For this review, use the dimensioned drawing (mm, ordinates from the lowest corner) and the shaded views. Round coordinates to 2 decimals unless told otherwise and drop trailing zeros. Write each loop counter-clockwise with the first axis right and the second up, starting at its lowest first coordinate (ties: lowest second). Pieces come first, ordered by that corner, then holes. Notation, with made-up numbers: (-27.5, 31.25) -> (-20.5, 31.25) arc R34 cw to (-20.5, 68.25) -> close; hole circle Ø10 at (-22, 18). An arc over 180 degrees is marked (long way). Answer as CSV lines item,"result". Start each with the question number.
Item 1: Take a section at C-C on y = 1.6. Give the boundary of the cut face in (x, z), then the cut area to 3 significant figures.
Item 2: For pin 1 Ø1.5 at (y, z) = (2.5, 34.5) entering from -X; pin 2 Ø1.5 at (x, y) = (6.5, 1.5) entering from -Z; pin 3 Ø1 at (y, z) = (2, 12) entering from -X; pin 4 Ø2.5 at (x, z) = (20, 5) entering from -Y, all flat-tipped, find the tip position at first contact; note any pin that passes through.
Item 3: Take a section at B-B on z = 5. Give the boundary of the cut face in (x, y).
Item 4: Take a section at D-D on z = 28.5. Give the boundary of the cut face in (x, y), then the cut area to 3 significant figures.
Item 5: Take a section at A-A on x = 20. Give the boundary of the cut face in (y, z).
Item 6: Wall thickness on probe 1 along Z at (x, y) = (20, 2.3); probe 2 along X at (y, z) = (2, 5); probe 3 along Z at (x, y) = (2.25, 2.8): over which ranges is each line inside the solid? List them lowest first. Write a range as from..to.
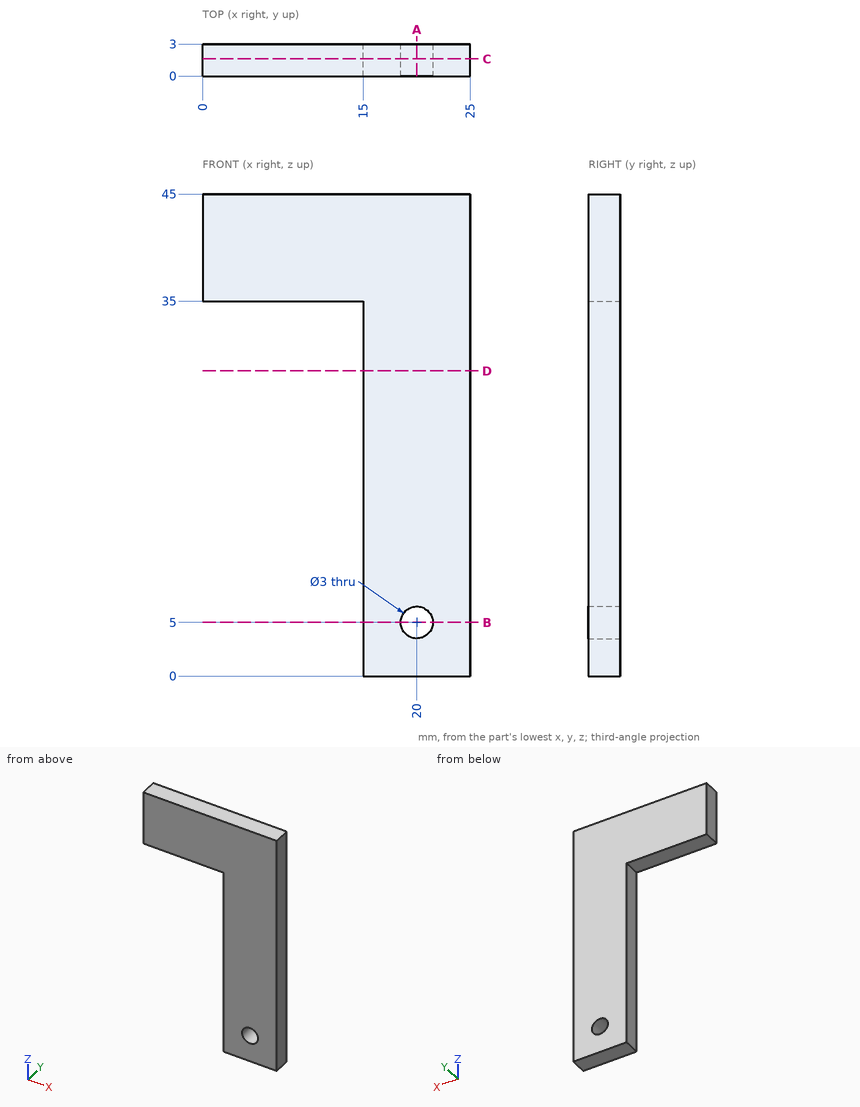
Output values:
1,outline,"(0, 35) -> (15, 35) -> (15, 0) -> (25, 0) -> (25, 45) -> (0, 45) -> close; hole circle Ø3 at (20, 5)"
1,area,"593 mm^2"
2,pin 1,"stops at x = 0"
2,pin 2,"stops at z = 35"
2,pin 3,"stops at x = 15"
2,pin 4,"passes through"
3,outline,"(15, 0) -> (18.5, 0) -> (18.5, 3) -> (15, 3) -> close; (21.5, 0) -> (25, 0) -> (25, 3) -> (21.5, 3) -> close"
4,outline,"(15, 0) -> (25, 0) -> (25, 3) -> (15, 3) -> close"
4,area,"30.0 mm^2"
5,outline,"(0, 0) -> (3, 0) -> (3, 3.5) -> (0, 3.5) -> close; (0, 6.5) -> (3, 6.5) -> (3, 45) -> (0, 45) -> close"
6,probe 1,"z = 0..3.5, 6.5..45"
6,probe 2,"x = 15..18.5, 21.5..25"
6,probe 3,"z = 35..45"
